Geometry check sheet. Reference: drawing and pictorial views, mm from the part's lowest x, y, z. Round coordinates to 2 decimals unless told otherwise and drop trailing zeros. Order: outer loops, then holes, each group sorted by start corner. A loop starts at its lowest first (then second) coordinate and runs counter-clockwise, first axis right, second up.
(1) Sectioned sample at A-A (z = 2.75). Record the boundary of the cut face in (x, y), plus the area to 3 significant figures.
(2) Sectioned sample at B-B (x = 166.5). Record the boundary of the cut face in (y, z), plus the area to 3 significant figures.
(3) Material ranges on line 1 along X through (y, z) = (13.25, 5.5); line 2 along X through (y, z) = (13, 5.25); line 3 along Y through (x, z) = (260, 7), recorded low to high.
(4) Go/stop test with flat-tipped pins: pin 1 (5 mm diameter, centred on x = 260, y = 10, fed in from +Z); pin 2 (3 mm diameter, centred on x = 146, z = 1, fed in from +Y). Record where each tip stops, or that it passes through.
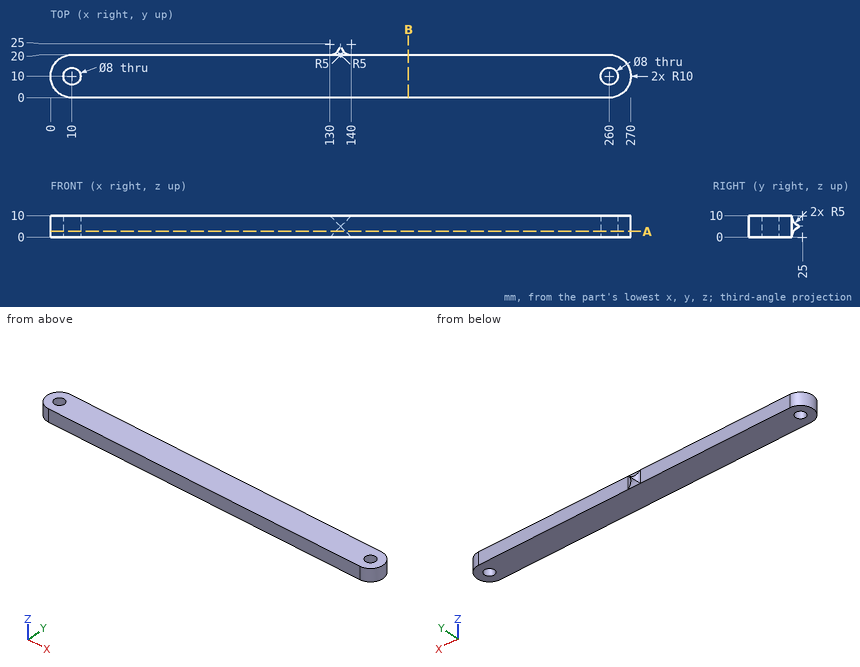
Answer below:
1. outline: (10, 0) - (260, 0) arc R10 ccw to (260, 20) - (140, 20) arc R5 cw to (137.25, 20.82) - (132.75, 20.82) arc R5 cw to (130, 20) - (10, 20) arc R10 ccw to start; hole circle Ø8 at (10, 10); hole circle Ø8 at (260, 10)
1. area: 5,220 mm2
2. outline: (0, 0) - (20, 0) - (20, 10) - (0, 10) - close
2. area: 200 mm2
3. line 1: x = 0.54 to 7.67, 12.33 to 257.67, 262.33 to 269.46
3. line 2: x = 0.46 to 7.35, 12.65 to 257.35, 262.65 to 269.54
3. line 3: y = 0 to 6, 14 to 20
4. pin 1: passes through
4. pin 2: stops at y = 20
